Autodesk Inventor part; units mm, degrees
ref_plane "YZ Plane" through (0, 0, 0) normal (1, 0, 0) x (0, 1, 0)
ref_plane "XZ Plane" through (0, 0, 0) normal (0, 1, 0) x (-1, 0, 0)
ref_plane "XY Plane" through (0, 0, 0) normal (0, 0, 1) x (1, 0, 0)
sketch "スケッチ1" plane through (0, 0, 0) normal (0, 1, 0) x (-1, 0, 0)
  circle A0 centre (0, 0) radius 57.5
  circle A1 centre (0, 0) radius 70
  dimension "d0" = 115
  dimension "d1" = 140
extrude "押し出し1" add sketch "スケッチ1" along normal blind 8.5
fillet "フィレット1" radius 1 2 edges at (57.5, 8.5, 0) (70, 8.5, 0)
sketch "スケッチ3" plane through (0, 8.5, 0) normal (0, 1, 0) x (1, 0, 0)
  circle A0 centre (0, 0) radius 64
  point P0 (0, 64)
  point P1 (64, 0)
  point P2 (0, -64)
  point P3 (-64, 0)
  dimension "d19" = 128
hole "穴2" at (0, 8.5, -64) at (64, 8.5, 0) at (0, 8.5, 64) at (-64, 8.5, 0) direction (0, -1, 0) diameter 5.1 end through all
properties part number "turntable_out_8_23" material "アルミニウム 6061-AHC"
Could you check a few things on this model? Use its own coordinates, in mm. Give positions to 0.01 mm unless a question says otherwise; leave off trailing zeros. Write each loop counter-clockwise with the first axis right and the second up, starting at its lowest first coordinate (ties: lowest second). Pieces come first, ordered by that corner, then holes. Notation, with made-up numbers: (78.25, -15) - (113.25, -15) arc R23 cw to (113.25, 21) - close; hole circle Ø7 at (-4.75, -29.5). An arc over 180 degrees is marked (long way). Use CSV: the item, a comma, the result in double quotes. Start each with the question number.
Item 1: If we mould it in two halves opening along X, with no side actions, what happens to faces 1 (the face through (55.55, 3.698, 42.594)), 2 (the face through (-0.112, 4.19, 61.452)), 3 (the face through (57, 8.5, -15))? For each: pulls with the +X half, pulls with the -X half, needs draft (parallel to the pull), parting line crosses it, or undercut.
Item 2: I'm going to push flat-ended pins straight in: pin 1 (4 mm diameter, centred on x = 0, z = 64, fed in from -Y); pin 2 (1.5 mm diameter, centred on y = 1, z = -9.5, fed in from -X); pin 3 (3 mm diameter, centred on x = 43, y = 4, fed in from +Z); pin 4 (1.5 mm diameter, centred on x = -10, y = 3, fed in from -Z). Where does each tip first touch, or does it pass through?
Item 3: If I drill on line 1 along Z through (x, y) = (0, 2.75); line 2 along Z through (x, y) = (-64, 5.25), over which ranges is the centre line in solid material (lowest first)?
Item 4: I want a section at A-A, the plane y = 5.5. Please give me the cut outline in (x, z).
Findings:
1,face 1,"parting line crosses it"
1,face 2,"undercut"
1,face 3,"needs draft"
2,pin 1,"passes through"
2,pin 2,"stops at x = -69.45"
2,pin 3,"stops at z = 56.37"
2,pin 4,"stops at z = -69.39"
3,line 1,"z = -70 to -66.55, -61.45 to -57.5, 57.5 to 61.45, 66.55 to 70"
3,line 2,"z = -28.35 to -2.55, 2.55 to 28.35"
4,outline,"circle Ø140 at (0, 0); hole circle Ø5.1 at (-64, 0); hole circle Ø115 at (0, 0); hole circle Ø5.1 at (0, -64); hole circle Ø5.1 at (0, 64); hole circle Ø5.1 at (64, 0)"
